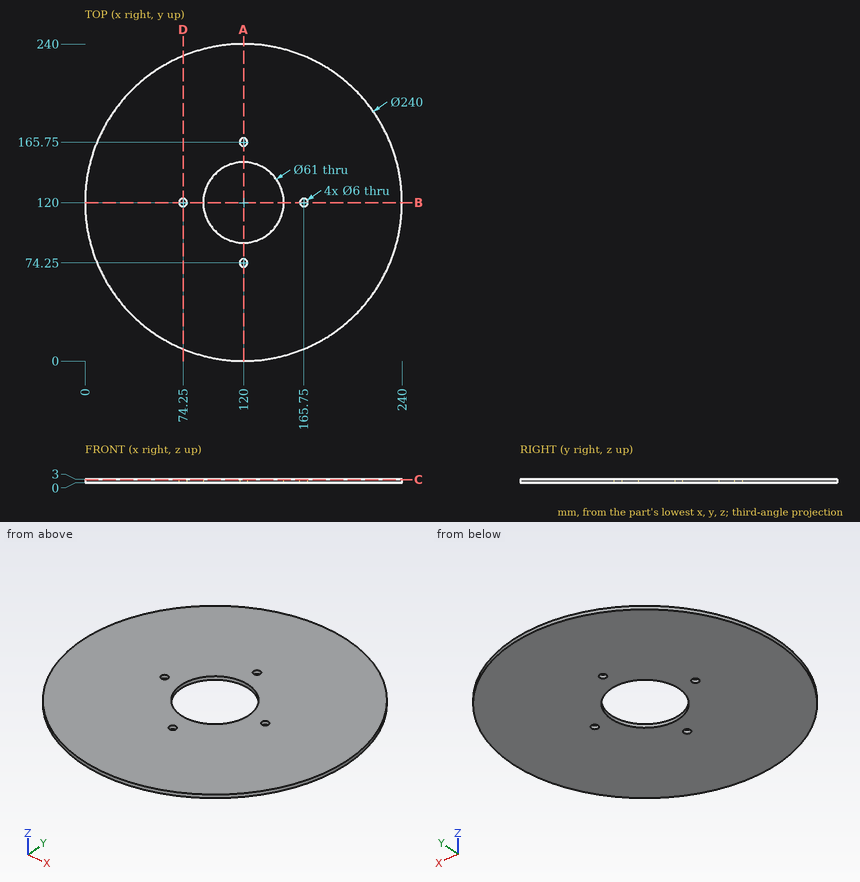
Input: dimensioned drawing with shaded views. Units: mm. Origin: part minimum x, y, z. Give positions to 0.01 mm unless a question says otherwise; leave off trailing zeros. Loops run counter-clockwise (first coordinate to the right, second up) from the corner with the lowest first, then second, coordinate; pieces in that order, holes last. Notation, with made-up numbers: (48, 79) -> (66, 79) arc R31 ccw to (66, 105) -> close; hole circle Ø6 at (65, 45.25). An arc over 180 degrees is marked (long way). Use a Markdown table: item, result.
Q1. Section query C-C, the plane z = 2.55. Return the cut outline in (x, y), plus the area to 3 significant figures.
Entries:
| item | result |
|---|---|
| outline | circle Ø240 at (120, 120); hole circle Ø6 at (74.25, 120); hole circle Ø61 at (120, 120); hole circle Ø6 at (120, 74.25); hole circle Ø6 at (120, 165.75); hole circle Ø6 at (165.75, 120) |
| area | 42,200 mm² |
Q2. First-contact query: P1, Ø9.5, axis at x = 120, y = 165.75, coming from the +Z side; P2, Ø1.5, axis at x = 168.5, z = 1, coming from the -Y side. Flat tips, straight axial feed; report the tip coordinate or a pass-through.
Entries:
| item | result |
|---|---|
| P1 | stops at z = 3 |
| P2 | stops at y = 9.91 |
Q3. Section query D-D, the plane x = 74.25. Return the cut outline in (y, z), plus the area to 3 significant figures.
Entries:
| item | result |
|---|---|
| outline | (9.06, 0) -> (117, 0) -> (117, 3) -> (9.06, 3) -> close; (123, 0) -> (230.94, 0) -> (230.94, 3) -> (123, 3) -> close |
| area | 648 mm² |
Q4. Section query A-A, the plane x = 120. Return the cut outline in (y, z), plus the area to 3 significant figures.
Entries:
| item | result |
|---|---|
| outline | (0, 0) -> (71.25, 0) -> (71.25, 3) -> (0, 3) -> close; (77.25, 0) -> (89.5, 0) -> (89.5, 3) -> (77.25, 3) -> close; (150.5, 0) -> (162.75, 0) -> (162.75, 3) -> (150.5, 3) -> close; (168.75, 0) -> (240, 0) -> (240, 3) -> (168.75, 3) -> close |
| area | 501 mm² |
Q5. Ray query, probe 1 along Y at (x, z) = (120, 0.9); probe 2 along Y at (x, z) = (117.5, 2.5); probe 3 along Y at (x, z) = (125.5, 0.5). Return the intervals inside material, ascending. Write a range as from..to.
Entries:
| item | result |
|---|---|
| probe 1 | y = 0..71.25, 77.25..89.5, 150.5..162.75, 168.75..240 |
| probe 2 | y = 0.03..72.59, 75.91..89.6, 150.4..164.09, 167.41..239.97 |
| probe 3 | y = 0.13..90, 150..239.87 |
